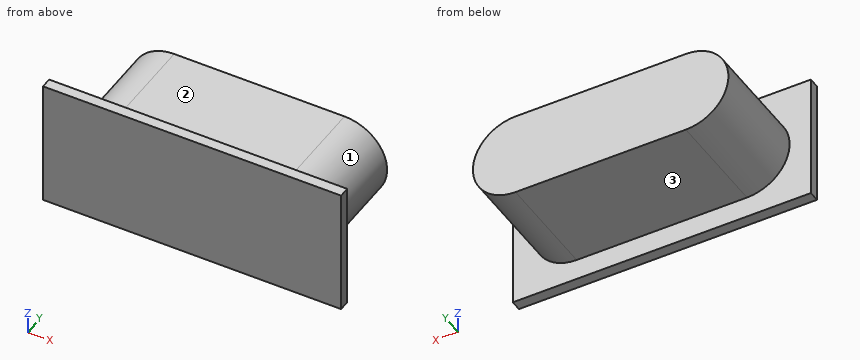
```python
from build123d import *

# Parameters (mm, degrees)
SKETCH1_W           = 7
SKETCH1_H           = 3
BOSS_EXTRUDE1_DEPTH = 0.25
BOSS_EXTRUDE2_DEPTH = 2.5


with BuildPart() as part:
    # Sketch1 → Boss-Extrude1 (new body)
    with BuildSketch(Plane(origin=(0, 0, 0), x_dir=(1, 0, 0), z_dir=(0, 1, 0))):
        Rectangle(SKETCH1_W, SKETCH1_H)
    extrude(amount=BOSS_EXTRUDE1_DEPTH)

    # Sketch2 → Boss-Extrude2 (add)
    with BuildSketch(Plane(origin=(0, 0.25, 0), x_dir=(1, 0, 0), z_dir=(0, 1, 0))):
        with BuildLine():
            Line((2, -1), (-2, -1))
            ThreePointArc((-2, -1), (-3, 0), (-2, 1))
            Line((-2, 1), (2, 1))
            ThreePointArc((2, 1), (3, 0), (2, -1))
        make_face()
    extrude(amount=BOSS_EXTRUDE2_DEPTH)


solid = part.part
```
For this review, take the finished solid that the model builds, in its own axes (mm). Face numbers are marked on the shaded views. A direction names the side the tool comes from. Coordinates: 2 decimals unless noted, no trailing zeros. Loops run counter-clockwise (first coordinate to the right, second up) from the corner with the lowest first, then second, coordinate; pieces in that order, holes last. Notation, with made-up numbers: (32.5, -36) - (77.5, -36) arc R22 cw to (77.5, -4) - close; hole circle Ø4 at (52.25, 82). An arc over 180 degrees is marked (long way). Use one line per item in the form item = value. Start each with the question number.
1) Take a section at C-C (y = 1.15). State the section outline as (x, z) points.
2) For pin 1 (1.5 mm diameter, centred on y = 1.5, z = 0.5, fed in from +X); pin 2 (1 mm diameter, centred on x = -2, y = 2, fed in from -Z), all flat-tipped, find the tip position at first contact; note any pin that passes through.
3) Take a section at D-D (z = 1.35). State the section outline as (x, y) points.
4) For the marked faces 1, 2 and 3, list the 3-axis set-ups (+Z, -Z, +X, -X, +Y, -Y) from which the entire face can be reached by the end or side of a thin tool; tool diameter is ignored.
5) Take a section at A-A (z = 0.8). State the section outline as (x, y) points.
6) Take a section at B-B (x = -0.25). State the section outline as (y, z) points.
7) To check wall thickness, follow probe 1 along Y at (x, z) = (-1.75, -1.1); probe 2 along Z at (x, y) = (1.75, 0.3); probe 3 along X at (y, z) = (0.6, -0.5). State the ranges of each line that lie inside material, in increasing order. Write a range as from..to.
From the geometry:
q1.outline = (-2, -1) - (2, -1) arc R1 ccw to (2, 1) - (-2, 1) arc R1 ccw to start
q2.pin_1 = 3
q2.pin_2 = -1
q3.outline = (-3.5, 0) - (3.5, 0) - (3.5, 0.25) - (-3.5, 0.25) - close
q4.face_1 = +X, +Y
q4.face_2 = +Z, +X, -X, +Y
q4.face_3 = -Z, +X, -X, +Y
q5.outline = (-3.5, 0) - (3.5, 0) - (3.5, 0.25) - (2.6, 0.25) - (2.6, 2.75) - (-2.6, 2.75) - (-2.6, 0.25) - (-3.5, 0.25) - close
q6.outline = (0, -1.5) - (0.25, -1.5) - (0.25, -1) - (2.75, -1) - (2.75, 1) - (0.25, 1) - (0.25, 1.5) - (0, 1.5) - close
q7.probe_1 = 0..0.25
q7.probe_2 = -1..1
q7.probe_3 = -2.87..2.87
